Design review of the part built by this model. Coordinates are the model's own, in mm. Give positions to 0.01 mm unless a question says otherwise; leave off trailing zeros. Order: outer loops, then holes, each group sorted by start corner. A loop starts at its lowest first (then second) coordinate and runs counter-clockwise, first axis right, second up. Notation, with made-up numbers: M 51.25,31.5 L 85.25,31.5 A30 cw 85.25,61.5 Z; hole C 57,73.25 d11. An arc over 180 degrees is marked long. Put each result on its own line as item: value. Start each with the question number.
from build123d import *

# Parameters (mm, degrees)
SKETCH1_W           = 2.54
SKETCH1_H           = 2.54
BOSS_EXTRUDE1_DEPTH = 8.52
SKETCH2_W           = 0.64
SKETCH2_H           = 0.64
CUT_EXTRUDE1_DEPTH  = 6.5
FILLET1_R           = 0.5
SKETCH4_W           = 0.5
SKETCH4_H           = 0.7
BOSS_EXTRUDE2_DEPTH = 3.18
SKETCH5_R           = 0.255
CUT_EXTRUDE4_DEPTH  = 0.26
SKETCH6_R           = 0.165430126
BOSS_EXTRUDE3_DEPTH = 0.1


with BuildPart() as part:
    # Sketch1 → Boss-Extrude1 (new body)
    with BuildSketch(Plane.XY):
        Rectangle(SKETCH1_W, SKETCH1_H)
    extrude(amount=BOSS_EXTRUDE1_DEPTH)

    # Sketch2 → Cut-Extrude1 (cut)
    with BuildSketch(Plane.XY.offset(8.52)):
        Rectangle(SKETCH2_W, SKETCH2_H)
    extrude(amount=-CUT_EXTRUDE1_DEPTH, mode=Mode.SUBTRACT)

    # Fillet1
    fillet1_edges = [part.edges().sort_by_distance(p)[0] for p in [
        (0.32, 0, 8.52),
        (0, 0.32, 8.52),
        (-0.32, 0, 8.52),
        (0, -0.32, 8.52),
    ]]
    fillet(fillet1_edges, radius=FILLET1_R)

    # Sketch4 → Boss-Extrude2 (add)
    with BuildSketch(Plane(origin=(0, 0, 0), x_dir=(1, 0, 0), z_dir=(0, 0, -1))):
        Rectangle(SKETCH4_W, SKETCH4_H)
    extrude(amount=BOSS_EXTRUDE2_DEPTH)

    # Sketch5 → Cut-Extrude4 (cut)
    with BuildSketch(Plane.XY.offset(2.02)):
        Circle(SKETCH5_R)
    extrude(amount=-CUT_EXTRUDE4_DEPTH, mode=Mode.SUBTRACT)

    # Sketch6 → Boss-Extrude3 (add)
    with BuildSketch(Plane(origin=(0, 0, -3.18), x_dir=(-1, 0, 0), z_dir=(0, 0, -1))):
        Circle(SKETCH6_R)
    extrude(amount=BOSS_EXTRUDE3_DEPTH)


solid = part.part
1. Consider section C-C on y = 0. Give the boundary of the cut face in (x, z) (3 decimals), then the cut area to 3 significant figures.
2. Consider section B-B on x = 0. Give the boundary of the cut face in (y, z) (3 decimals).
3. Insertion check: pin 1 (0.6 mm diameter, centred on x = 0, z = -1, fed in from +Y); pin 2 (0.6 mm diameter, centred on y = 0, z = -2, fed in from -X); pin 3 (0.6 mm diameter, centred on y = 0, z = -1, fed in from +X). Each pin has a flat end and moves straight along its axis. Give the tip position at first contact, or say it passes through.
4. To check wall thickness, follow probe 1 along Y at (x, z) = (0, 1.8) (3 decimals); probe 2 along X at (y, z) = (-0.25, 3); probe 3 along Z at (x, y) = (0.3, -0.8). State the ranges of each line that lie inside material, in increasing order.
5. Consider section A-A on z = 6. Give the boundary of the cut face in (x, y).
6. Consider section D-D on y = 0.45. Give the boundary of the cut face in (x, z), then the cut area to 3 significant figures.
Returned:
1. outline: M -1.27,0 L -0.25,0 L -0.25,-3.18 L -0.165,-3.18 L -0.165,-3.28 L 0.165,-3.28 L 0.165,-3.18 L 0.25,-3.18 L 0.25,0 L 1.27,0 L 1.27,8.52 L 0.82,8.52 A0.5 ccw 0.32,8.02 L 0.32,2.02 L 0.255,2.02 L 0.255,1.76 L -0.255,1.76 L -0.255,2.02 L -0.32,2.02 L -0.32,8.02 A0.5 ccw -0.82,8.52 L -1.27,8.52 Z
1. area: 18.9 mm2
2. outline: M -1.27,0 L -0.35,0 L -0.35,-3.18 L -0.165,-3.18 L -0.165,-3.28 L 0.165,-3.28 L 0.165,-3.18 L 0.35,-3.18 L 0.35,0 L 1.27,0 L 1.27,8.52 L 0.82,8.52 A0.5 ccw 0.32,8.02 L 0.32,2.02 L 0.255,2.02 L 0.255,1.76 L -0.255,1.76 L -0.255,2.02 L -0.32,2.02 L -0.32,8.02 A0.5 ccw -0.82,8.52 L -1.27,8.52 Z
3. pin 1: stops at y = 0.35
3. pin 2: stops at x = -0.25
3. pin 3: stops at x = 0.25
4. probe 1: y = -1.27 to -0.255, 0.255 to 1.27
4. probe 2: x = -1.27 to -0.32, 0.32 to 1.27
4. probe 3: z = 0 to 8.52
5. outline: M -1.27,-1.27 L 1.27,-1.27 L 1.27,1.27 L -1.27,1.27 Z; hole M -0.32,-0.32 L 0.32,-0.32 L 0.32,0.32 L -0.32,0.32 Z
6. outline: M -1.27,0 L 1.27,0 L 1.27,8.52 L 0.82,8.52 A0.5 ccw 0.45,8.36 L -0.45,8.36 A0.5 ccw -0.82,8.52 L -1.27,8.52 Z
6. area: 21.5 mm2
